Can you work these out from the model? Positions are in its coordinate system, mm. A direction names the side the tool comes from. Round coordinates to 2 decimals unless told otherwise and drop trailing zeros. Loops run counter-clockwise (first coordinate to the right, second up) from the corner with the lowest first, then second, coordinate; pieces in that order, holes last. Notation, with made-up numbers: (37.25, -40) -> (76.25, -40) arc R16 ccw to (76.25, -20) -> close; hole circle Ø4 at (14.25, 42.5). An arc over 180 degrees is marked (long way). Write each question's results on one line, items separated by ' | '.
from build123d import *

# Parameters (mm, degrees)
SKETCH_R        = 4.575
PAD_DEPTH       = 1.7
SKETCH001_R     = 2.375
PAD001_DEPTH    = 45
CHAMFER_SIZE2   = 2.25
CHAMFER_SIZE    = 0.15
POCKET_DEPTH    = 2.5
CHAMFER001_SIZE = 0.25
FILLET_R        = 0.5


with BuildPart() as part:
    # Sketch → Pad (new body)
    with BuildSketch(Plane.XZ):
        Circle(SKETCH_R)
    extrude(amount=PAD_DEPTH)

    # Sketch001 (on Face3 of Pad) → Pad001 (join)
    with BuildSketch(Plane.XZ.offset(1.7)):
        Circle(SKETCH001_R)
    extrude(amount=PAD001_DEPTH)

    # Chamfer
    chamfer_edges = [part.edges().sort_by_distance(p)[0] for p in [
        (-2.375, -1.7, 0),
    ]]
    chamfer_side = part.faces().sort_by_distance((-4.445599, -1.7, 0))[0]
    chamfer(chamfer_edges, length=CHAMFER_SIZE, length2=CHAMFER_SIZE2, reference=chamfer_side)

    # Sketch002 (on Face5 of Chamfer) → Pocket (cut)
    with BuildSketch(Plane(origin=(0, 0, 0), x_dir=(-1, 0, 0), z_dir=(0, 1, 0))):
        Polygon((1.732051, 1), (0, 2), (-1.732051, 1), (-1.732051, -1), (0, -2), (1.732051, -1), align=None)
    extrude(amount=-POCKET_DEPTH, mode=Mode.SUBTRACT)

    # Chamfer001
    chamfer001_edges = [part.edges().sort_by_distance(p)[0] for p in [
        (-1.732051, 0, 0),
        (-0.866025, 0, 1.5),
        (0.866025, 0, 1.5),
        (1.732051, 0, 0),
        (0.866025, 0, -1.5),
        (-0.866025, 0, -1.5),
    ]]
    chamfer(chamfer001_edges, length=CHAMFER001_SIZE)

    # Fillet
    fillet_edges = [part.edges().sort_by_distance(p)[0] for p in [
        (4.575, -0.85, 0),
        (-4.575, 0, 0),
        (-4.575, -1.7, 0),
    ]]
    fillet(fillet_edges, radius=FILLET_R)


solid = part.part
1. On a 3-axis mill with a long thin cutter (end or side, diameter ignored), from which of +Z, -Z, +X, -X, +Y, -Y can I reach the whole of each face in a straight line? I mean faces 1 (the face through (1.096, -25.026, -2.107)), 2 (the face through (0, -46.7, 0)), 3 (the face through (-0.85, -1.36, -1.51)). Say none if no direction works.
Final values:
face 1: -Y | face 2: +Z, -Z, +X, -X, -Y | face 3: +Y
2. Will these pins go through, and if not, where does the flat tip stop? pin 1 (5 mm diameter, centred on y = -12.5, z = 2.5, fed in from -X) (3 decimals); pin 2 (2 mm diameter, centred on y = -29.5, z = 3, fed in from +X); pin 3 (5 mm diameter, centred on y = -29, z = -1.5, fed in from +X) (3 decimals).
Final values:
pin 1: x = -2.375 | pin 2: x = 1.28 | pin 3: x = 2.375
3. If we section it at B-B (y = -27): List the corners of the cut face in (x, z) for me (3 decimals).
Final values:
outline: circle Ø4.75 at (0, 0)
4. If we section it at A-A (z = 0): List the corners of the cut face in (x, y) for me (3 decimals).
Final values:
outline: (-4.575, -1.2) arc R0.5 ccw to (-4.075, -1.7) -> (-2.525, -1.7) -> (-2.375, -3.95) -> (-2.375, -46.7) -> (2.375, -46.7) -> (2.375, -3.95) -> (2.525, -1.7) -> (4.075, -1.7) arc R0.5 ccw to (4.575, -1.2) -> (4.575, -0.5) arc R0.5 ccw to (4.075, 0) -> (1.982, 0) -> (1.732, -0.25) -> (1.732, -2.5) -> (-1.732, -2.5) -> (-1.732, -0.25) -> (-1.982, 0) -> (-4.075, 0) arc R0.5 ccw to (-4.575, -0.5) -> close
5. Please list where these lines run through material, in increasing order: line 1 (Y direction, x = 0.25, z = 3); line 2 (Y direction, x = 1.5, z = -1); line 3 (Z direction, x = 0.5, y = -10.5). Write a range as from..to.
Final values:
line 1: -1.7..0 | line 2: -46.7..-2.5 | line 3: -2.32..2.32
